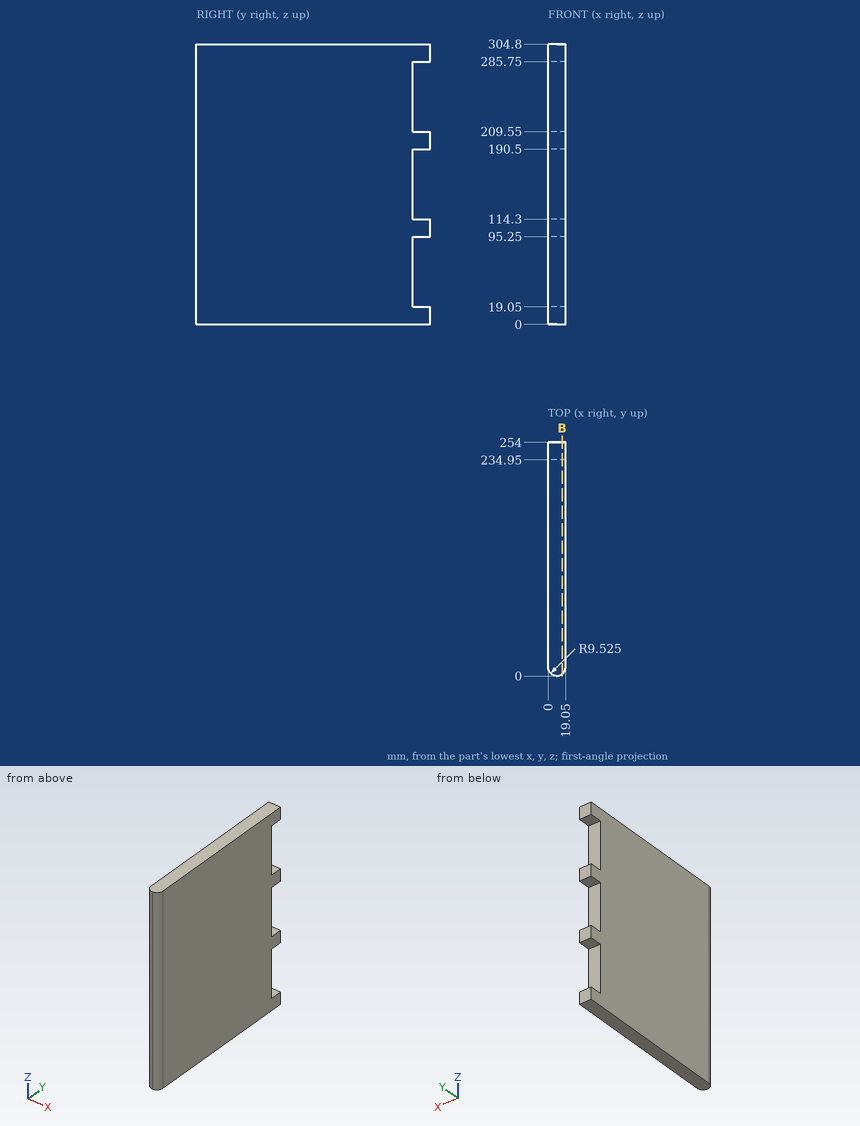
Part print with two shaded views. Sizes in mm from the minimum x, y, z corner. Round coordinates to 2 decimals unless told otherwise and drop trailing zeros. Write each loop counter-clockwise with the first axis right and the second up, starting at its lowest first coordinate (ties: lowest second). Pieces come first, ordered by that corner, then holes. Notation, with made-up numbers: M 75,58.5 L 90,58.5 A12 cw 90,68.5 Z; hole C 18,-23 d9. An arc over 180 degrees is marked long. Put each result on its own line as item: value. Start each with the question number.
1) Pin check, flat tips, straight feed: pin 1 Ø9.5 at (x, z) = (11.5, 166.5) entering from +Y; pin 2 Ø9.5 at (x, y) = (14, 240.5) entering from -Z; pin 3 Ø4 at (x, z) = (7, 71) entering from -Y. Stop position of each tip, or through.
2) Drill centre lines: probe 1 along Z at (x, y) = (9, 239.5); probe 2 along Y at (x, z) = (8.5, 37); probe 3 along Y at (x, z) = (9, 291). Where is each one in solid material? Low to high. Write a range as [from, to].
3) Saw through at B-B, the plane x = 15.25. Write the cut outline in (y, z).
Resolved:
1. pin 1: y = 234.95
1. pin 2: z = 0
1. pin 3: y = 0.01
2. probe 1: [0, 19.05], [95.25, 114.3], [190.5, 209.55], [285.75, 304.8]
2. probe 2: [0.06, 234.95]
2. probe 3: [0.01, 254]
3. outline: M 1.91,0 L 254,0 L 254,19.05 L 234.95,19.05 L 234.95,95.25 L 254,95.25 L 254,114.3 L 234.95,114.3 L 234.95,190.5 L 254,190.5 L 254,209.55 L 234.95,209.55 L 234.95,285.75 L 254,285.75 L 254,304.8 L 1.91,304.8 Z
